Part model, mm, in its own coordinate system. A direction names the side the tool comes from. Give positions to 0.01 mm unless a question says otherwise; leave off trailing zeros. Write each loop counter-clockwise with the first axis right and the second up, starting at its lowest first coordinate (ties: lowest second). Pieces come first, ordered by that corner, then holes. Notation, with made-up numbers: M 1,0 L 28,0 A20 cw 28,13 Z; hole C 44.5,60.5 d6. An arc over 180 degrees is marked long. Use a Markdown table: item, result. Add a question column.
from build123d import *

# Parameters (mm, degrees)
F2_T     = -5.08
F3_R     = 63.5
F4_DEPTH = 781.3280539866
F6_DEPTH = 254
F7_COUNT = 24


with BuildPart() as f1:
    # F0 (on Front) → F1 (revolve)
    with BuildSketch(Plane.XZ):
        Polygon((-673.1, 0), (0, 0), (0, 781.3270539866), (-127, 781.3270539866), (-127, 400.3270539866), (-673.1, 254), align=None)
    revolve(axis=Axis((0, 0, 390.6635269933), (0, 0, -1)))

    # F2
    f2_openings = [f1.faces().sort_by_distance(p)[0] for p in [
        (0, 0, 0),
    ]]
    offset(amount=F2_T, openings=f2_openings, kind=Kind.INTERSECTION)

    # F3 (on Top) → F4 (cut, through all)
    with BuildSketch(Plane.XY):
        Circle(F3_R)
    extrude(amount=F4_DEPTH, mode=Mode.SUBTRACT)

    # F5 (on face) → F6 (join)
    with BuildSketch(Plane(origin=(0, 0, 0), x_dir=(1, 0, 0), z_dir=(0, 0, -1))):
        with BuildLine():
            ThreePointArc((-671.1830188679, -50.7638176592), (-673.1, 0), (-671.1830188679, 50.7638176592))
            ThreePointArc((-671.1830188679, 50.7638176592), (-723.9, 0), (-671.1830188679, -50.7638176592))
        make_face()
    extrude(amount=-F6_DEPTH)

    # F7: F1 ×24 about axis
    f7_axis = Axis((0, 0, 781.3270539866), (0, 0, -1))


with BuildPart() as f1_1:
    add(f1.part)
    for i in range(1, F7_COUNT):
        add(f1.part.rotate(f7_axis, i * 360 / F7_COUNT))


solid = f1_1.part
1. Drill centre lines: probe 1 along Y at (x, z) = (0, 588); probe 2 along Y at (x, z) = (0, 779.3); probe 3 along Y at (x, z) = (-513.5, 139.5). Where is each one in solid material? Low to high. Write a range as [from, to].
2. Flat gauge pins, fed straight in: pin 1 (16 mm diameter, centred on x = -10.5, y = 692.5, fed in from +Z); pin 2 (10 mm diameter, centred on x = -503, y = -426.5, fed in from -Z); pin 3 (3 mm diameter, centred on x = -279, y = -531.5, fed in from -Z). Where does each tip first touch, or does it go through?
3. Cut at B-B (z = 611.5). Write the cut outline in (x, y).
4. Cut at A-A (x = 0). Write the cut outline in (y, z).
5. Tool access for faces 1 (the cylindrical face through (86.963, 662.335, 123.3)), 2 (the cylindrical face through (-362.934, 626.333, 125.222)), 3 (the flat face through (-347, 599, 254)), 4 (the flat face through (-345, -600, 254)), 5 (the flat face through (489, 490, 254)): list every direction of +Z, -Z, +X, -X, +Y, -Y with a clear straight run to the whole face (end or side of a thin tool).
6. Mould opens along Y. For faces 6 (the cylindrical face through (-699.517, 186.251, 125.222)), 7 (the cylindrical face through (-87.34, -667.41, 125.22)), 8 (the flat face through (-669, 178, 254)), 9 (the cylindrical face through (-627.48, 360.95, 125.22)) say: released by +Y, released by -Y, zero draft, split by the parting line, or undercut.
A:
| question | item | result |
|---|---|---|
| 1 | probe 1 | y = [-127, -121.92], [121.92, 127] |
| 1 | probe 2 | y = [-127, -63.5], [63.5, 127] |
| 1 | probe 3 | y = [-510.17, -441.74], [-435.18, -427.28], [427.28, 435.18], [441.74, 510.17] |
| 2 | pin 1 | stops at z = 254 |
| 2 | pin 2 | stops at z = 251.05 |
| 2 | pin 3 | stops at z = 267.85 |
| 3 | outline | C 0,0 d254; hole C 0,0 d243.84 |
| 4 | outline | M -723.9,0 L -668.02,0 L -668.02,250.1 L -121.92,396.43 L -121.92,776.25 L -63.5,776.25 L -63.5,781.33 L -127,781.33 L -127,400.33 L -673.1,254 L -723.9,254 Z; M 63.5,776.25 L 121.92,776.25 L 121.92,396.43 L 668.02,250.1 L 668.02,0 L 723.9,0 L 723.9,254 L 673.1,254 L 127,400.33 L 127,781.33 L 63.5,781.33 Z |
| 5 | face 1 | -Z |
| 5 | face 2 | +Z, -Z |
| 5 | face 3 | +Z, -X, +Y |
| 5 | face 4 | +Z, -X, -Y |
| 5 | face 5 | +Z, +X, +Y |
| 6 | face 6 | undercut |
| 6 | face 7 | released by -Y |
| 6 | face 8 | zero draft |
| 6 | face 9 | undercut |
